Solid Edge part; units mm, degrees
sketch "Sketch1" plane through (0, 0, 0) normal (0, -1, 0) x (1, 0, 0)
  line L0 (0, 0) -> (0, 6)
  arc A0 (0, 6) -> (5, 6) centre (2.5, 6) cw
  line L1 (5, 6) -> (5, 0)
  arc A1 (0, 0) -> (5, 0) centre (2.5, 0) ccw
extrude "Protrusion1" add sketch "Sketch1" against normal blind 2
sketch "Sketch2" plane through (5, 1, 3) normal (1, 0, 0) x (0, 1, 0)
  line L0 (1, 5.5) -> (0.25, 5.5)
  arc A0 (0.25, 5.5) -> (0.25, -5.5) centre (11.725, 0) ccw
  line L1 (1, -5.5) -> (0.25, -5.5)
  line L2 (1, 5.5) -> (1, -5.5)
extrude "ExtrudedCutout_1" cut sketch "Sketch2" against normal blind 43.2268 flip side to cut
sketch "Sketch3" plane through (2.5, 0, 3) normal (0, -1, 0) x (0, 0, 1)
  arc A0 (-3, 2) -> (-3, -2) centre (-3, 0) ccw
  line L0 (-3, -2) -> (3, -2)
  arc A1 (3, 2) -> (3, -2) centre (3, 0) cw
  line L1 (-3, 2) -> (3, 2)
extrude "ExtrudedCutout_2" cut sketch "Sketch3" against normal blind 1.25
sketch "Sketch4" plane through (2.5, 2, 3) normal (0, 1, 0) x (0, 0, 1)
  circle A0 centre (0, 0) radius 1.25
  circle A1 centre (0, 0) radius 1.35
extrude "ExtrudedProtrusion_2" add sketch "Sketch4" along normal blind 0.25
sketch "Sketch5" plane through (2.5, 2, 3) normal (0, 1, 0) x (0, 0, 1)
  arc A0 (-3, 2.15) -> (-3, -2.15) centre (-3, 0) ccw
  line L0 (-3, -2.15) -> (3, -2.15)
  arc A1 (3, -2.15) -> (3, 2.15) centre (3, 0) ccw
  line L1 (3, 2.15) -> (-3, 2.15)
  arc A2 (-3, 2.5) -> (-3, -2.5) centre (-3, 0) ccw
  line L2 (-3, -2.5) -> (3, -2.5)
  arc A3 (3, -2.5) -> (3, 2.5) centre (3, 0) ccw
  line L3 (3, 2.5) -> (-3, 2.5)
extrude "ExtrudedProtrusion_4" add sketch "Sketch5" along normal blind 0.25
properties material "Stainless Steel, 420"
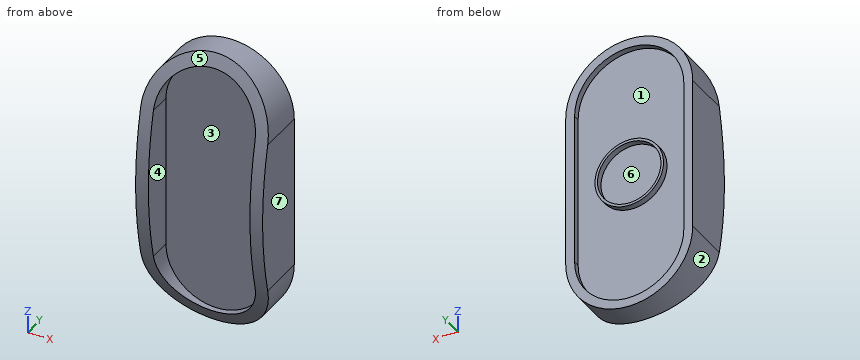
The model under review builds one solid part; all positions refer to its coordinate system, in mm. Face numbers are marked on the shaded views. A direction names the side the tool comes from. Round coordinates to 2 decimals unless told otherwise and drop trailing zeros. Write each loop counter-clockwise with the first axis right and the second up, starting at its lowest first coordinate (ties: lowest second). Pieces come first, ordered by that corner, then holes. Notation, with made-up numbers: (-32.5, 46.25) - (-28.5, 46.25) arc R25 cw to (-28.5, 76.25) - close; hole circle Ø1 at (0.25, 1). An arc over 180 degrees is marked (long way). One line per item, written item: value. Start each with the question number.
1. Clearance check with flat-ended pins moving along their axes: P1, Ø2, axis at x = 2.5, z = 3, coming from the +Y side; P2, Ø1, axis at x = 4, y = 0.5, coming from the -Z side; P3, Ø1, axis at x = 4, y = 1, coming from the +Z side. State where each tip first meets the part, or that it passes through.
2. Consider section A-A on y = 0.2. Write out the cut boundary in (x, z), and give its area (3 significant figures).
3. Consider section B-B on z = 3. Write out the cut boundary in (x, y).
4. The part is to be moulded in two halves that separate along Z. For the marked faces 4, 5, 6 and 7, say which applies: released by +Z, released by -Z, zero draft, split by the parting line, or undercut.
5. Machinability: for the marked faces 1, 2 and 3, which of the approach directions +Z, -Z, +X, -X, +Y, -Y give a long, thin tool a straight path to every point of the face, cutting with its end or side? Answer none if there is none.
6. Consider section D-D on x = 1.6. Write out the cut boundary in (y, z) (3 decimals), and give its area (3 significant figures).
7. To check wall thickness, follow L1, parallel to Y at x = 1.9, z = 0.25; L2, parallel to Z at x = 3.85, y = 1.1; L3, parallel to Z at x = 4.05, y = 2.05. State the ranges of each line that lie inside material, in increasing order. Write a range as from..to.
8. Consider section C-C on y = 1.15. Write out the cut boundary in (x, z), and give its area (3 significant figures).
Checks:
1. P1: stops at y = 2
1. P2: stops at z = -1.94
1. P3: stops at z = 8.28
2. outline: (0, 0.75) - (0.5, 0.75) - (0.5, 5.25) - (0, 5.25) - close; (4.5, 0.75) - (5, 0.75) - (5, 5.25) - (4.5, 5.25) - close
2. area: 4.49 mm^2
3. outline: (0, 0) - (0.5, 0) - (0.5, 1.25) - (4.5, 1.25) - (4.5, 0) - (5, 0) - (5, 2.25) - (4.65, 2.25) - (4.65, 2) - (3.85, 2) - (3.85, 2.25) - (3.75, 2.25) - (3.75, 2) - (1.25, 2) - (1.25, 2.25) - (1.15, 2.25) - (1.15, 2) - (0.35, 2) - (0.35, 2.25) - (0, 2.25) - close
4. face 4: undercut
4. face 5: split by the parting line
4. face 6: undercut
4. face 7: zero draft
5. face 1: +Y
5. face 2: -Z, +Y, -Y
5. face 3: -Y
6. outline: (0.934, -1.786) arc R12.725 ccw to (1.171, -2.332) - (2.25, -2.332) - (2.25, -1.953) - (2, -1.953) - (2, 1.994) - (2.25, 1.994) - (2.25, 2.133) - (2, 2.133) - (2, 3.867) - (2.25, 3.867) - (2.25, 4.006) - (2, 4.006) - (2, 7.953) - (2.25, 7.953) - (2.25, 8.332) - (1.171, 8.332) arc R12.725 ccw to (0.934, 7.786) - (1.25, 7.786) - (1.25, -1.786) - close
6. area: 8.48 mm^2
7. L1: y = 1.25..2
7. L2: z = -2.1..-1.48, 7.48..8.1
7. L3: z = -1.96..-1.49, 7.49..7.96
8. outline: (0, 0) arc R2.5 ccw to (1.49, -2.29) - (3.51, -2.29) arc R2.5 ccw to (5, 0) - (5, 6) arc R2.5 ccw to (3.51, 8.29) - (1.49, 8.29) arc R2.5 ccw to (0, 6) - close; hole (0.5, 0) arc R2 ccw to (4.5, 0) - (4.5, 6) arc R2 ccw to (0.5, 6) - close
8. area: 12.5 mm^2
